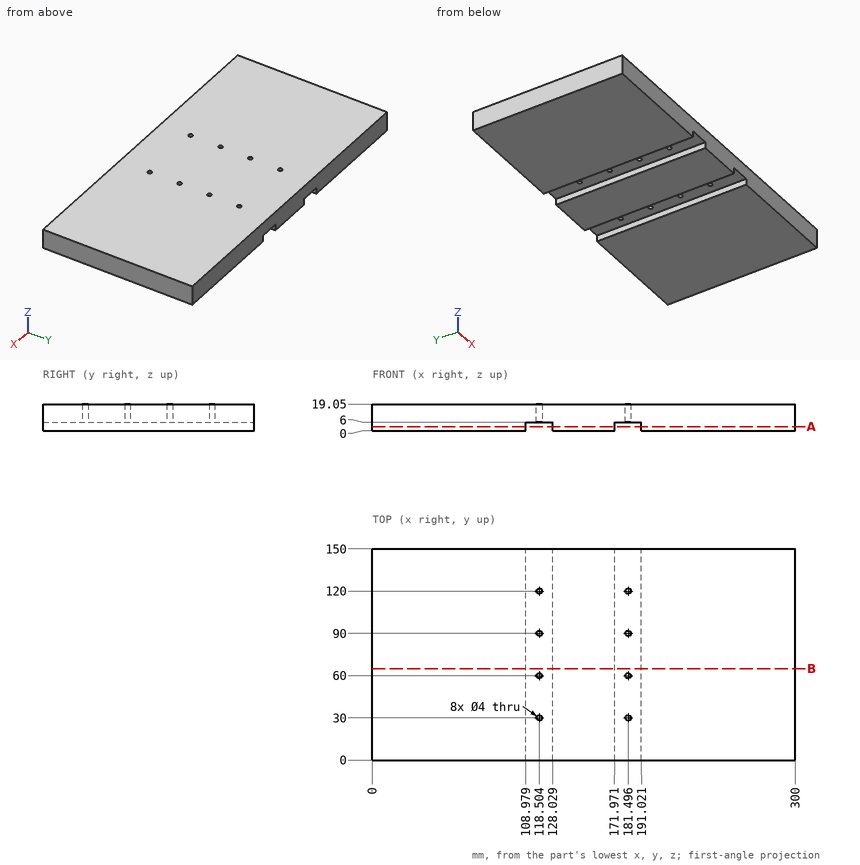
Verification items for this drawing (mm, ordinates from the low corner). Coordinates: 2 decimals unless noted, no trailing zeros. Loops run counter-clockwise (first coordinate to the right, second up) from the corner with the lowest first, then second, coordinate; pieces in that order, holes last. Notation, with made-up numbers: (-30, -39) - (-21, -39) arc R6 cw to (-21, -29) - close; hole circle Ø7 at (-24.5, 27.5). An arc over 180 degrees is marked (long way). One line per item, written item: value. Start each with the question number.
(1) Material ranges on line 1 (X direction, y = 59, z = 5); line 2 (Z direction, x = 122.5, y = 38.5), recorded low to high. Write a range as [from, to].
(2) Cross-section at B-B on y = 65. Enter the section's corners in (x, z).
(3) Cross-section at A-A on z = 3. Enter the section's corners in (x, y), plus the area to 3 significant figures.
(4) Depth check by flat-ended pin: P1, Ø4.5, axis at x = 118.504, y = 60, coming from the -Z side. Enter the tip coordinate at first touch or a pass-through.
Results below:
1. line 1: x = [0, 108.98], [128.03, 171.97], [191.02, 300]
1. line 2: z = [6, 19.05]
2. outline: (0, 0) - (108.98, 0) - (108.98, 6) - (128.03, 6) - (128.03, 0) - (171.97, 0) - (171.97, 6) - (191.02, 6) - (191.02, 0) - (300, 0) - (300, 19.05) - (0, 19.05) - close
3. outline: (0, 0) - (108.98, 0) - (108.98, 150) - (0, 150) - close; (128.03, 0) - (171.97, 0) - (171.97, 150) - (128.03, 150) - close; (191.02, 0) - (300, 0) - (300, 150) - (191.02, 150) - close
3. area: 39,300 mm2
4. P1: stops at z = 6
